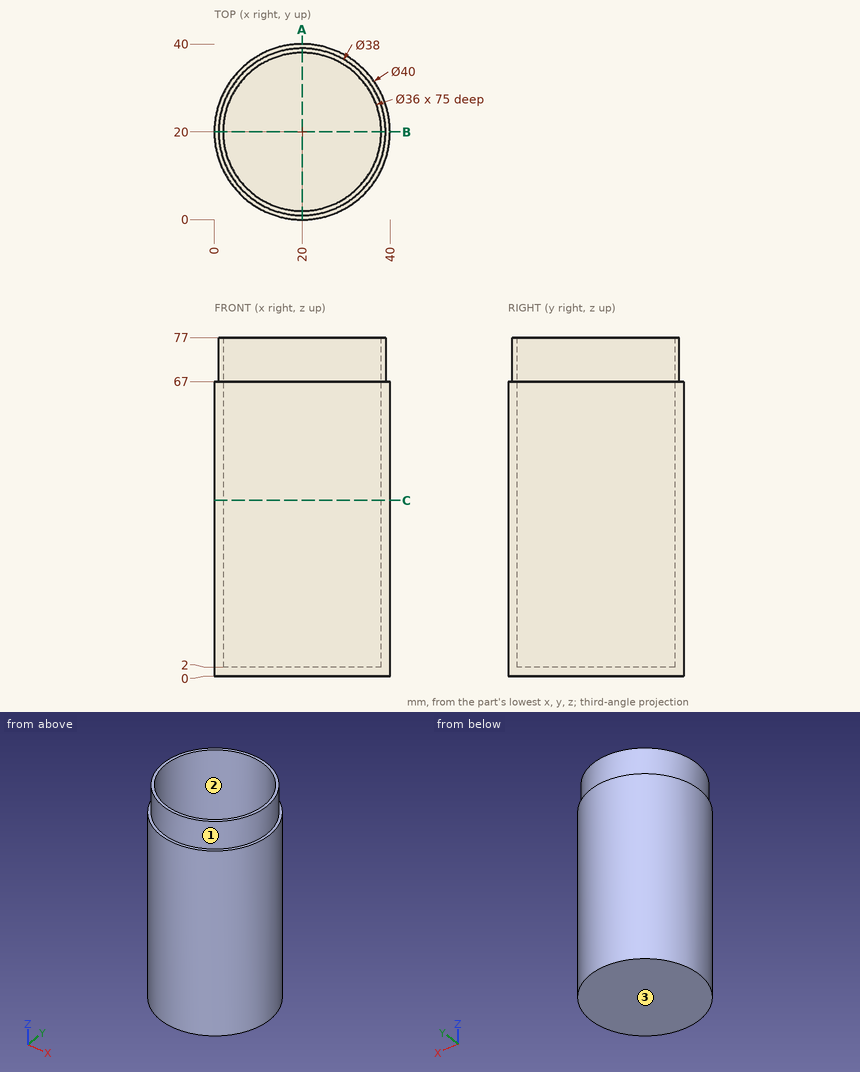
Source: three-view drawing plus pictorial views. Frame: mm from the lowest corner of the part. Round coordinates to 2 decimals unless told otherwise and drop trailing zeros. Loops run counter-clockwise (first coordinate to the right, second up) from the corner with the lowest first, then second, coordinate; pieces in that order, holes last.
Q1. Section A-A, the plane x = 20. Return loops of the section in (y, z).
Q2. Ray query, line 1 (Z direction, x = 16.5, y = 11); line 2 (Y direction, x = 20, z = 30); line 3 (Y direction, x = 8, z = 26.5). Return the intervals inside material, ascending.
Q3. Mould query, pull axis X, two halves, no side actions, for the marked faces 1, 2 and 3. Classes: pulls with the +X half, pulls with the -X half, needs draft (parallel to the pull), parting line crosses it, or undercut.
Q4. First-contact query: P1, Ø2, axis at y = 30, z = 48.5, coming from the -X side; P2, Ø1, axis at x = 4, z = 42.5, coming from the +Y side; P3, Ø6, axis at x = 14.5, z = 13, coming from the +Y side. Flat tips, straight axial feed; report the tip coordinate or a pass-through.
Q5. Section C-C, the plane z = 40. Return loops of the section in (x, y).
Solutions:
1. outline: (0, 0) - (40, 0) - (40, 67) - (39, 67) - (39, 77) - (38, 77) - (38, 2) - (2, 2) - (2, 77) - (1, 77) - (1, 67) - (0, 67) - close
2. line 1: z = 0 to 2
2. line 2: y = 0 to 2, 38 to 40
2. line 3: y = 4 to 6.58, 33.42 to 36
3. face 1: parting line crosses it
3. face 2: undercut
3. face 3: needs draft
4. P1: stops at x = 2.14
4. P2: stops at y = 32.64
4. P3: stops at y = 39.84
5. outline: circle Ø40 at (20, 20); hole circle Ø36 at (20, 20)
